Geometry: final body of the model. Coordinates: model frame, mm. A direction names the side the tool comes from. Give positions to 0.01 mm unless a question says otherwise; leave off trailing zeros. Order: outer loops, then holes, each group sorted by start corner. A loop starts at its lowest first (then second) coordinate and runs counter-clockwise, first axis right, second up. Notation, with made-up numbers: (-31, 63.25) - (-19, 63.25) arc R8 ccw to (-19, 71.25) - close; hole circle Ø7 at (-19.5, 62.25). An arc over 180 degrees is marked (long way). One line per question, with ' | ' between items. Start each with the question number.
from build123d import *

# Parameters (mm, degrees)
SKETCH1_W               = 100
SKETCH1_H               = 290
BOSS_EXTRUDE1_DEPTH     = 6
SKETCH2_W               = 62
SKETCH2_H               = 26
CUT_EXTRUDE1_DEPTH      = 7
SKETCH3_W               = 52
SKETCH3_H               = 290
CUT_EXTRUDE2_DEPTH      = 2
SKETCH4_R               = 2.5
SKETCH4_R_2             = 5.25
SKETCH4_R_3             = 2.1
SKETCH4_R_4             = 3.3
CUT_EXTRUDE_HOLES_DEPTH = 21
FILLET1_R               = 3
FILLET2_R               = 6
CHAMFER1_SIZE           = 2
SKETCH5_R               = 5.75
CUT_EXTRUDE5_DEPTH      = 5
CHAMFER2_SIZE           = 2
CHAMFER3_SIZE           = 0.3


with BuildPart() as part:
    # Sketch1 → Boss-Extrude1 (new, symmetric)
    with BuildSketch(Plane.XY):
        Rectangle(SKETCH1_W, SKETCH1_H)
    extrude(amount=BOSS_EXTRUDE1_DEPTH, both=True)

    # Sketch2 → Cut-Extrude1 (cut)
    with BuildSketch(Plane.XY.offset(6)):
        with Locations((0, 132)):
            Rectangle(SKETCH2_W, SKETCH2_H)
    extrude(amount=-CUT_EXTRUDE1_DEPTH, mode=Mode.SUBTRACT)

    # Sketch3 → Cut-Extrude2 (cut)
    with BuildSketch(Plane.XY.offset(6)):
        Rectangle(SKETCH3_W, SKETCH3_H)
    extrude(amount=-CUT_EXTRUDE2_DEPTH, mode=Mode.SUBTRACT)

    # Sketch4 → Cut-Extrude HOLES (cut)
    with BuildSketch(Plane.XY.offset(-6)):
        with Locations((-23, 139)):
            Circle(SKETCH4_R)
        with Locations((23, 139)):
            Circle(SKETCH4_R)
        with Locations((23, 126)):
            Circle(SKETCH4_R)
        with Locations((-23, 126)):
            Circle(SKETCH4_R)
        with Locations(Location((0, 57.59, 0), (0, 0, 180))):
            Circle(SKETCH4_R_2)
        with Locations(Location((-18, 83.89, 0), (0, 0, 180))):
            Circle(SKETCH4_R_3)
        with Locations(Location((-18, 57.59, 0), (0, 0, 180))):
            Circle(SKETCH4_R_4)
        with Locations(Location((-18, 35.09, 0), (0, 0, 180))):
            Circle(SKETCH4_R_4)
        with Locations((-36, 70)):
            Circle(SKETCH4_R_3)
        with Locations((-36, 10)):
            Circle(SKETCH4_R_3)
        with Locations((-36, -110)):
            Circle(SKETCH4_R_3)
        with Locations((-36, -50)):
            Circle(SKETCH4_R_3)
        with Locations(Location((-18, -103.65, 0), (0, 0, 180))):
            Circle(SKETCH4_R_4)
        with Locations(Location((-18, -126.15, 0), (0, 0, 180))):
            Circle(SKETCH4_R_4)
        with Locations(Location((18, -103.65, 0), (0, 0, 180))):
            Circle(SKETCH4_R_4)
        with Locations(Location((18, -126.15, 0), (0, 0, 180))):
            Circle(SKETCH4_R_4)
        with Locations(Location((0, -133.65, 0), (0, 0, 180))):
            Circle(SKETCH4_R_4)
        with Locations(Location((36, 70, 0), (0, 0, 180))):
            Circle(SKETCH4_R_3)
        with Locations(Location((18, 83.89, 0), (0, 0, 180))):
            Circle(SKETCH4_R_3)
        with Locations(Location((18, 35.09, 0), (0, 0, 180))):
            Circle(SKETCH4_R_4)
        with Locations(Location((18, 57.59, 0), (0, 0, 180))):
            Circle(SKETCH4_R_4)
        with Locations(Location((36, 10, 0), (0, 0, 180))):
            Circle(SKETCH4_R_3)
        with Locations(Location((36, -50, 0), (0, 0, 180))):
            Circle(SKETCH4_R_3)
        with Locations(Location((36, -110, 0), (0, 0, 180))):
            Circle(SKETCH4_R_3)
    extrude(amount=CUT_EXTRUDE_HOLES_DEPTH, mode=Mode.SUBTRACT)

    # Fillet1
    fillet1_edges = [part.edges().sort_by_distance(p)[0] for p in [
        (-31, 119, 2.5),
        (31, 119, 2.5),
    ]]
    fillet(fillet1_edges, radius=FILLET1_R)

    # Fillet2
    fillet2_edges = [part.edges().sort_by_distance(p)[0] for p in [
        (-50, 145, 0),
        (50, 145, 0),
    ]]
    fillet(fillet2_edges, radius=FILLET2_R)

    # Chamfer1
    chamfer1_edges = [part.edges().sort_by_distance(p)[0] for p in [
        (50, -3, 6),
        (-37.5, 145, 6),
        (37.5, 145, 6),
        (48.242640687, 143.242640687, 6),
        (-50, -3, 6),
        (-48.242640687, 143.242640687, 6),
    ]]
    chamfer(chamfer1_edges, length=CHAMFER1_SIZE)

    # Sketch5 → Cut-Extrude5 (cut)
    with BuildSketch(Plane.XY.offset(4)):
        with Locations((-18, 57.59)):
            Circle(SKETCH5_R)
        with Locations((-18, 35.09)):
            Circle(SKETCH5_R)
        with Locations((18, 35.09)):
            Circle(SKETCH5_R)
        with Locations((18, 57.59)):
            Circle(SKETCH5_R)
        with Locations((18, -103.65)):
            Circle(SKETCH5_R)
        with Locations((-18, -103.65)):
            Circle(SKETCH5_R)
        with Locations((-18, -126.15)):
            Circle(SKETCH5_R)
        with Locations((0, -133.65)):
            Circle(SKETCH5_R)
        with Locations((18, -126.15)):
            Circle(SKETCH5_R)
    extrude(amount=-CUT_EXTRUDE5_DEPTH, mode=Mode.SUBTRACT)

    # Chamfer2
    chamfer2_edges = [part.edges().sort_by_distance(p)[0] for p in [
        (5.25, 57.59, 4),
    ]]
    chamfer(chamfer2_edges, length=CHAMFER2_SIZE)

    # Chamfer3
    chamfer3_edges = [part.edges().sort_by_distance(p)[0] for p in [
        (0, 145, -6),
        (-50, -3, -6),
        (-48.242640687, 143.242640687, -6),
        (48.242640687, 143.242640687, -6),
        (50, -3, -6),
    ]]
    chamfer(chamfer3_edges, length=CHAMFER3_SIZE)


solid = part.part
(1) Access query for faces 1 (the cylindrical face through (-23.744, 35.343, 1.535)), 2 (the cylindrical face through (-2.42, 62.25, -2.06)), 3 (the flat face through (0, 132, -1)). Directions: +Z, -Z, +X, -X, +Y, -Y. A direction counts if a zero-diameter tool reaches every point of the face in a straight line with its end or side. Return the directions, or none.
(2) Cut plane A-A, the plane y = 35.09. Return the cut outline in (x, z).
(3) Pull-direction query (Y, two-part tool) for faces 4 (the cylindrical face through (16.754, 51.977, 1.535)), 5 (the flat face through (31, 133, 3)), 6 (the flat face through (0, 119, 2)); classes: +Y half, -Y half, draft (parallel to the pull), parting line (faces both ways), or undercut.
(4) Material intervals for line 1 along Y through (x, z) = (18, -2.1); line 2 along Y through (x, z) = (0, 0.75); line 3 along Y through (x, z) = (-18, 2.7), sorted ascending. Write a range as from..to.
(5) Contact query for flat-ended pins moving along their axis: P1, Ø12.5, axis at x = 19, y = 55, coming from the +Z side; P2, Ø3.5, axis at x = 19.5, y = -124, coming from the +Z side; P3, Ø2.5, axis at x = 36, y = 10, coming from the -Z side. Output: stop coordinate, or through.
(6) Cut plane B-B, the plane y = -5.5. Return the cut outline in (x, z), plus the area to 3 significant figures.
Results are:
1) face 1: +Z | face 2: +Z, -Z | face 3: +Z, +Y
2) outline: (-50, -5.7) - (-49.7, -6) - (-21.3, -6) - (-21.3, -1) - (-23.75, -1) - (-23.75, 4) - (-26, 4) - (-26, 6) - (-48, 6) - (-50, 4) - close; (-14.7, -6) - (14.7, -6) - (14.7, -1) - (12.25, -1) - (12.25, 4) - (-12.25, 4) - (-12.25, -1) - (-14.7, -1) - close; (21.3, -6) - (49.7, -6) - (50, -5.7) - (50, 4) - (48, 6) - (26, 6) - (26, 4) - (23.75, 4) - (23.75, -1) - (21.3, -1) - close
3) face 4: undercut | face 5: draft | face 6: +Y half
4) line 1: -145..-129.45, -122.85..-106.95, -100.35..31.79, 38.39..54.29, 60.89..81.79, 85.99..145 | line 2: -145..-139.4, -127.9..52.34, 62.84..119 | line 3: -145..-131.9, -120.4..-109.4, -97.9..29.34, 40.84..51.84, 63.34..81.79, 85.99..119
5) P1: z = 4 | P2: z = -1 | P3: through
6) outline: (-50, -5.7) - (-49.7, -6) - (49.7, -6) - (50, -5.7) - (50, 4) - (48, 6) - (26, 6) - (26, 4) - (-26, 4) - (-26, 6) - (-48, 6) - (-50, 4) - close | area: 1,090 mm2
